Check sheet for the modelled part. Datum: model origin and axes. Units: mm. Face numbers are marked on the shaded views. Round coordinates to 2 decimals unless told otherwise and drop trailing zeros. Write each loop counter-clockwise with the first axis right and the second up, starting at its lowest first coordinate (ties: lowest second). Pieces come first, ordered by that corner, then holes.
Item 1: Section check D-D, the plane y = 66. Record the cut outline in (x, z), plus the area to 3 significant figures.
Item 2: Release check for a two-part mould opening along X. For the marked faces 1, 2 and 3 record: pulls with the +X half, pulls with the -X half, needs draft (parallel to the pull), parting line crosses it, or undercut.
Item 3: Section check A-A, the plane z = -46.5. Record the cut outline in (x, y).
Item 4: Material ranges on line 1 along X through (y, z) = (78, -448); line 2 along Z through (x, y) = (464.5, 18); line 3 along Y through (x, z) = (92.5, -144), recorded low to high.
Item 5: Section check C-C, the plane x = 257. Record the cut outline in (y, z).
Item 6: Section check B-B, the plane x = 47.5. Record the cut outline in (y, z), plus the area to 3 significant figures.
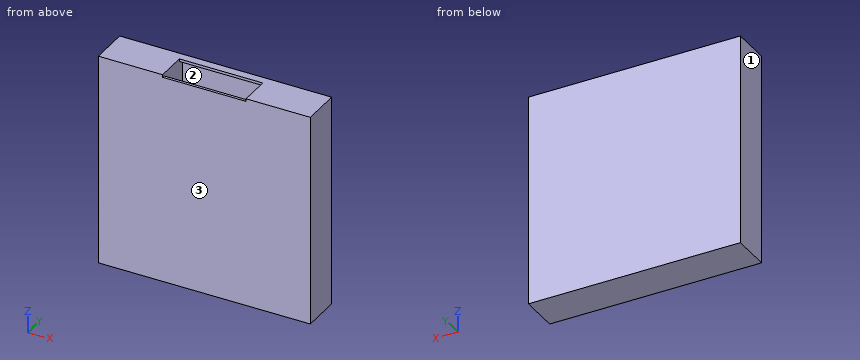
from build123d import *

# Parameters (mm, degrees)
SKETCH3_W               = 508
SKETCH3_H               = 508
BOSS_EXTRUDE1_DEPTH     = 6.3
SKETCH4_W               = 508
SKETCH4_H               = 508
SKETCH4_W_2             = 495.4
SKETCH4_H_2             = 495.4
BOSS_EXTRUDE2_DEPTH     = 80
SKETCH5_W               = 508
SKETCH5_H               = 508
BOSS_EXTRUDE3_DEPTH     = 6.3
SKETCH6_W               = 200
SKETCH6_H               = 72.6
CUT_EXTRUDE2_DEPTH      = 1
CUT_EXTRUDE2_DEPTH_BACK = 6.3
SKETCH8_W               = 6.3
SKETCH8_H               = 92.6
BOSS_EXTRUDE4_DEPTH     = 508


with BuildPart() as part:
    # Sketch3 → Boss-Extrude1 (new body)
    with BuildSketch(Plane(origin=(0, 0, 0), x_dir=(1, 0, 0), z_dir=(0, 1, 0))):
        with Locations((254, 254)):
            Rectangle(SKETCH3_W, SKETCH3_H)
    extrude(amount=BOSS_EXTRUDE1_DEPTH)

    # Sketch4 → Boss-Extrude2 (add)
    with BuildSketch(Plane(origin=(0, 6.3, 0), x_dir=(1, 0, 0), z_dir=(0, 1, 0))):
        with Locations((254, 254)):
            Rectangle(SKETCH4_W, SKETCH4_H)
        with Locations((254, 254)):
            Rectangle(SKETCH4_W_2, SKETCH4_H_2, mode=Mode.SUBTRACT)
    extrude(amount=BOSS_EXTRUDE2_DEPTH)

    # Sketch5 → Boss-Extrude3 (add)
    with BuildSketch(Plane(origin=(0, 86.3, 0), x_dir=(1, 0, 0), z_dir=(0, 1, 0))):
        with Locations((254, 254)):
            Rectangle(SKETCH5_W, SKETCH5_H)
    extrude(amount=BOSS_EXTRUDE3_DEPTH)

    # Sketch6 → Cut-Extrude2 (cut, two sides)
    with BuildSketch(Plane.XY) as cut_extrude2_sk:
        with Locations((254, 36.3)):
            Rectangle(SKETCH6_W, SKETCH6_H)
    extrude(amount=CUT_EXTRUDE2_DEPTH, mode=Mode.SUBTRACT)
    extrude(cut_extrude2_sk.sketch, amount=-CUT_EXTRUDE2_DEPTH_BACK, mode=Mode.SUBTRACT)

    # Sketch8 → Boss-Extrude4 (add)
    with BuildSketch(Plane.XY):
        with Locations((150.85, 46.3)):
            Rectangle(SKETCH8_W, SKETCH8_H)
        with Locations((357.15, 46.3)):
            Rectangle(SKETCH8_W, SKETCH8_H)
    extrude(amount=-BOSS_EXTRUDE4_DEPTH)


solid = part.part
Values found:
1. outline: (0, -508) - (508, -508) - (508, 0) - (354, 0) - (354, -501.7) - (154, -501.7) - (154, 0) - (0, 0) - close; hole (6.3, -501.7) - (147.7, -501.7) - (147.7, -6.3) - (6.3, -6.3) - close; hole (360.3, -501.7) - (501.7, -501.7) - (501.7, -6.3) - (360.3, -6.3) - close
1. area: 17,600 mm2
2. face 1: pulls with the -X half
2. face 2: undercut
2. face 3: needs draft
3. outline: (0, 0) - (508, 0) - (508, 92.6) - (0, 92.6) - close; hole (6.3, 6.3) - (147.7, 6.3) - (147.7, 86.3) - (6.3, 86.3) - close; hole (154, 6.3) - (354, 6.3) - (354, 86.3) - (154, 86.3) - close; hole (360.3, 6.3) - (501.7, 6.3) - (501.7, 86.3) - (360.3, 86.3) - close
4. line 1: x = 0 to 6.3, 147.7 to 154, 354 to 360.3, 501.7 to 508
4. line 2: z = -508 to -501.7, -6.3 to 0
4. line 3: y = 0 to 6.3, 86.3 to 92.6
5. outline: (0, -508) - (92.6, -508) - (92.6, 0) - (72.6, 0) - (72.6, -6.3) - (86.3, -6.3) - (86.3, -501.7) - (6.3, -501.7) - (6.3, -6.3) - (0, -6.3) - close
6. outline: (0, -508) - (92.6, -508) - (92.6, 0) - (0, 0) - close; hole (6.3, -501.7) - (86.3, -501.7) - (86.3, -6.3) - (6.3, -6.3) - close
6. area: 7,410 mm2
